The listing builds one solid part. Answer for the finished solid, in the listing's coordinates (mm). Face numbers are marked on the shaded views. A direction names the side the tool comes from. Give positions to 0.01 mm unless a question says otherwise; leave off trailing zeros. Write each loop counter-clockwise with the first axis right and the second up, starting at its lowest first coordinate (ties: lowest second). Pieces come first, ordered by that corner, then holes. Notation, with made-up numbers: (85, 56.5) - (136, 56.5) arc R17 cw to (136, 77.5) - close; hole circle Ø3 at (-10.5, 35). An arc over 180 degrees is marked (long way). Answer in a Markdown table with one row per item. Add a question column.
from build123d import *

# Parameters (mm, degrees)
SKETCH_1_R          = 24
EXTRUDE_1_DEPTH     = 8
SKETCH_2_R          = 16
EXTRUDE_2_DEPTH     = 8
SKETCH_4_R          = 5
SKETCH_4_R_2        = 4
SKETCH_4_R_3        = 2
CUT_EXTRUDE_1_DEPTH = 38.523326079


with BuildPart() as part:
    # 草图1 → 凸台-拉伸1 (new body)
    with BuildSketch(Plane(origin=(0, 0, 0), x_dir=(1, 0, 0), z_dir=(0, 1, 0))):
        with Locations(Location((0, 0, 0), (0, 0, 270))):
            Circle(SKETCH_1_R)
    extrude(amount=EXTRUDE_1_DEPTH)

    # 草图2 → 凸台-拉伸2 (add)
    with BuildSketch(Plane(origin=(0, 8, 0), x_dir=(1, 0, 0), z_dir=(0, 1, 0))):
        with Locations(Location((0, 0, 0), (0, 0, 270))):
            Circle(SKETCH_2_R)
    extrude(amount=EXTRUDE_2_DEPTH)

    # 草图4 → 切除-拉伸1 (cut, through all)
    with BuildSketch(Plane(origin=(0, 16, 0), x_dir=(1, 0, 0), z_dir=(0, 1, 0))):
        with Locations(Location((-10, 0, 0), (0, 0, 270))):
            Circle(SKETCH_4_R)
        with Locations(Location((0, 8, 0), (0, 0, 270))):
            Circle(SKETCH_4_R_2)
        with Locations(Location((0, -8, 0), (0, 0, 270))):
            Circle(SKETCH_4_R_2)
        with Locations(Location((10, 0, 0), (0, 0, 270))):
            Circle(SKETCH_4_R_3)
    extrude(amount=-CUT_EXTRUDE_1_DEPTH, mode=Mode.SUBTRACT)


solid = part.part
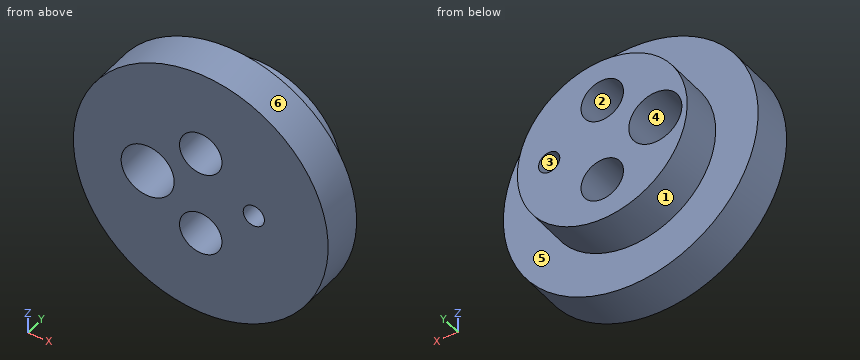
1. Section B-B (x = -6) is taken. Give the vertices of the cut face in (y, z), and give its area (3 significant figures).
2. The mould has two halves that part along X. Classify the marked faces 3, 4, 5 and 6: +X half, -X half, draft (parallel to the pull), parting line (faces both ways), or undercut.
3. Given pin 1 Ø1.5 at (x, y) = (-9.5, 5.5) entering from +Z; pin 2 Ø13 at (x, z) = (0, 8) entering from +Y; pin 3 Ø2 at (y, z) = (13.5, 4) entering from -X; pin 4 Ø2 at (x, y) = (-10.5, 9.5) entering from -Z, each flat-ended and moving along its own axis, determine where each tip first touches the part or whether it passes through.
4. Straight lines are drawn through the part: L1, parallel to X at y = 7.5, z = 0; L2, parallel to Z at x = -2.5, y = 4.25; L3, parallel to Z at x = -2.5, y = 8.75. For each, find the intervals that lie inside material, in ascending order. Write a range as [from, to].
5. Section A-A (z = 0) is taken. Give the vertices of the cut face in (x, y).
6. Section D-D (z = 7.5) is taken. Give the vertices of the cut face in (x, y), and give its area (3 significant figures).
7. Section C-C (y = 14) is taken. Give the vertices of the cut face in (x, z), and give its area (3 significant figures).
8. A tool of negligible diameter and unlimited length cuts with its end or side. For the marked faces 1 and 2, from which of +Z, -Z, +X, -X, +Y, -Y can it reach the whole face along a straight path? Write none if from no direction.
Geometry check:
| question | item | result |
|---|---|---|
| 1 | outline | (0, -23.24) - (8, -23.24) - (8, -14.83) - (16, -14.83) - (16, -3) - (0, -3) - close; (0, 3) - (16, 3) - (16, 14.83) - (8, 14.83) - (8, 23.24) - (0, 23.24) - close |
| 1 | area | 513 mm² |
| 2 | face 3 | undercut |
| 2 | face 4 | undercut |
| 2 | face 5 | draft |
| 2 | face 6 | parting line |
| 3 | pin 1 | z = 22.35 |
| 3 | pin 2 | y = 16 |
| 3 | pin 3 | x = -15.72 |
| 3 | pin 4 | z = -12.87 |
| 4 | L1 | [-24, -15], [-5, 8], [12, 24] |
| 4 | L2 | [-23.87, -11.12], [-4.88, 4.88], [11.12, 23.87] |
| 4 | L3 | [-15.8, -11.12], [-4.88, 4.88], [11.12, 15.8] |
| 5 | outline | (-24, 0) - (-15, 0) - (-15, 16) - (-16, 16) - (-16, 8) - (-24, 8) - close; (-5, 0) - (8, 0) - (8, 16) - (-5, 16) - close; (12, 0) - (24, 0) - (24, 8) - (16, 8) - (16, 16) - (12, 16) - close |
| 6 | outline | (-22.8, 0) - (-3.97, 0) - (-3.97, 16) - (-14.13, 16) - (-14.13, 8) - (-22.8, 8) - close; (3.97, 0) - (22.8, 0) - (22.8, 8) - (14.13, 8) - (14.13, 16) - (3.97, 16) - close |
| 6 | area | 464 mm² |
| 7 | outline | circle Ø32 at (0, 0); hole circle Ø10 at (-10, 0); hole circle Ø8 at (0, -8); hole circle Ø8 at (0, 8); hole circle Ø4 at (10, 0) |
| 7 | area | 613 mm² |
| 8 | face 1 | +Y |
| 8 | face 2 | +Y, -Y |
